```python
from build123d import *

# Parameters (mm, degrees)
PAD006_DEPTH           = 32
SKETCH014_R            = 6
POCKET004_DEPTH        = 232.94305
LINEARPATTERN002_COUNT = 4
LINEARPATTERN002_PITCH = 130


with BuildPart() as part:
    # Sketch013 → Pad006 (new body)
    with BuildSketch(Plane.XY):
        Polygon((-385.479931, 291.7), (10.181459, 14.654912), (6.74, 9.74), (-388.92139, 286.785088), align=None)
    extrude(amount=PAD006_DEPTH)

    # Sketch014 (on Face3 of Pad006) → Pocket004 (cut, through all)
    with BuildSketch(Plane(origin=(6.793695, 9.702402, 0), x_dir=(0.819152, -0.573576, 0), z_dir=(-0.573576, -0.819152, 0))):
        with Locations((-462.664681, 16)):
            Circle(SKETCH014_R)
    pocket004 = extrude(amount=-POCKET004_DEPTH, mode=Mode.SUBTRACT)

    # LinearPattern002: Pocket004 ×4
    with Locations(*[Vector(0.819152, -0.573576, 0) * (i * LINEARPATTERN002_PITCH) for i in range(1, LINEARPATTERN002_COUNT)]):
        add(pocket004, mode=Mode.SUBTRACT)


with BuildPart() as part_1:
    # Body005 placement: moved
    add(part.part.moved(Location((0, 0, 9))))


solid = part_1.part
```
Geometry: final body of the model. Coordinates: model frame, mm. Round coordinates to 2 decimals unless told otherwise and drop trailing zeros. Write each loop counter-clockwise with the first axis right and the second up, starting at its lowest first coordinate (ties: lowest second). Pieces come first, ordered by that corner, then holes.
Item 1: Section query A-A (y = 239.5). Return loops of the section in (x, z).
Item 2: Mould query, pull axis Z, two halves, no side actions, for faces 1 (the face through (-190.42, 155.12, 24.78)), 2 (the face through (-267.91, 205.67, 21.35)), 3 (the face through (-188, 151, 9)). Classes: +Z half, -Z half, draft (parallel to the pull), parting line (faces both ways), or undercut.
Item 3: Pin query (flat end, axial travel): P1, Ø1.5, axis at y = 253, z = 16.5, coming from the -X side; P2, Ø12, axis at y = 171, z = 15, coming from the +X side; P3, Ø12, axis at y = 52, z = 15.5, coming from the -X side. Return the tip coordinate at first contact, or that it passes through.
Item 4: Section query B-B (x = -25). Return loops of the section in (y, z), plus the area to 3 significant figures.
Item 5: Material intervals for L1, parallel to X at y = 57.5, z = 38.5; L2, parallel to Y at x = -82, z = 22.5; L3, parallel to Y at x = -155.5, z = 37, sorted ascending.
Completed:
1. outline: (-321.39, 9) - (-310.93, 9) - (-310.93, 41) - (-321.39, 41) - close
2. face 1: draft
2. face 2: undercut
2. face 3: -Z half
3. P1: stops at x = -341.74
3. P2: stops at x = -204.53
3. P3: stops at x = -62.18
4. outline: (31.96, 9) - (39.29, 9) - (39.29, 41) - (31.96, 41) - close
4. area: 234 mm2
5. L1: x = -61.47 to -51.01
5. L2: y = 71.88 to 79.2
5. L3: y = 123.34 to 130.67
